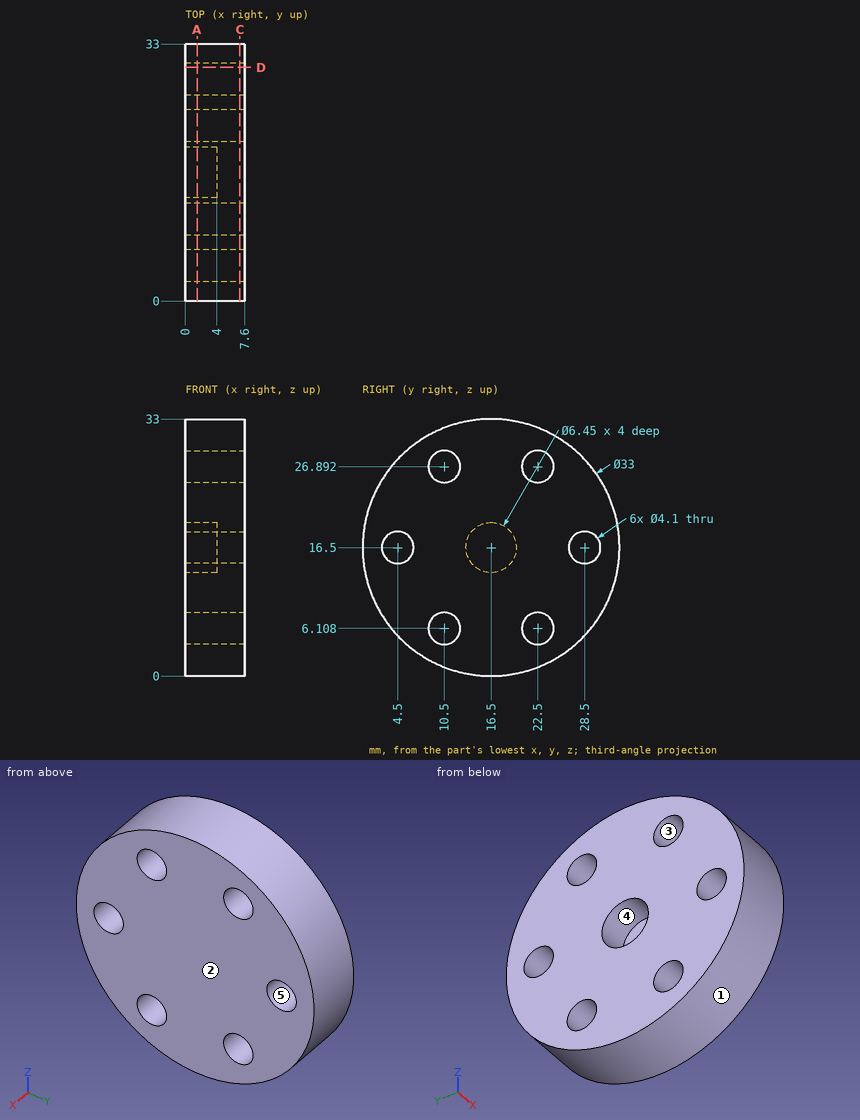
Verification items for this drawing (mm, ordinates from the low corner). A direction names the side the tool comes from. Coordinates: 2 decimals unless noted, no trailing zeros. Write each loop counter-clockwise with the first axis right and the second up, starting at its lowest first coordinate (ties: lowest second). Pieces come first, ordered by that corner, then holes. Notation, with made-up numbers: M 46.25,48.5 L 82.25,48.5 A34 cw 82.25,87.5 Z; hole C 14.5,1.25 d3. An arc over 180 degrees is marked long. Use one line per item in the form item = value. Start each with the question number.
1) Release check for a two-part mould opening along Y. For the marked faces 1, 2 and 3 record: pulls with the +Y half, pulls with the -Y half, needs draft (parallel to the pull), parting line crosses it, or undercut.
2) Section check C-C on x = 7. Enter the section's corners in (y, z), and give its area (3 significant figures).
3) Thickness scan on probe 1 along Y at (x, z) = (5, 16.5); probe 2 along Z at (x, y) = (4.75, 22.5); probe 3 along Y at (x, z) = (6.75, 5.5). Record the ranges inside material, lowest first. Write a range as from..to.
4) Go/stop test with flat-tipped pins: pin 1 Ø3 at (y, z) = (15.5, 16.5) entering from -X; pin 2 Ø2.5 at (y, z) = (10.5, 26.89) entering from +X; pin 3 Ø4 at (x, y) = (3, 27) entering from +Z; pin 4 Ø3 at (x, y) = (3.5, 29) entering from -Z. Record where each tip stops, or that it passes through.
5) Section check A-A on x = 1.5. State how many separate pieces and enclosed holes the cut face has.
6) Section check D-D on y = 30. Enter the section's corners in (x, z), and give its area (3 significant figures).
7) Set-up check for the marked faces 4 and 5: record each of +Z, -Z, +X, -X, +Y, -Y from which the full face is reachable in a straight line by a thin tool's end or side.
Responses:
q1.face_1 = parting line crosses it
q1.face_2 = needs draft
q1.face_3 = undercut
q2.outline = C 16.5,16.5 d33; hole C 4.5,16.5 d4.1; hole C 10.5,6.11 d4.1; hole C 10.5,26.89 d4.1; hole C 22.5,6.11 d4.1; hole C 22.5,26.89 d4.1; hole C 28.5,16.5 d4.1
q2.area = 776 mm2
q3.probe_1 = 0..2.45, 6.55..26.45, 30.55..33
q3.probe_2 = 1.13..4.06, 8.16..24.84, 28.94..31.87
q3.probe_3 = 4.2..8.54, 12.46..20.54, 24.46..28.8
q4.pin_1 = 4
q4.pin_2 = through
q4.pin_3 = 30.64
q4.pin_4 = 4.2
q5.separate_pieces = 1
q5.enclosed_holes = 7
q6.outline = M 0,7.01 L 7.6,7.01 L 7.6,15.1 L 0,15.1 Z; M 0,17.9 L 7.6,17.9 L 7.6,25.99 L 0,25.99 Z
q6.area = 123 mm2
q7.face_4 = -X
q7.face_5 = +X, -X
